Check sheet for the modelled part. Datum: model origin and axes. Units: mm. A direction names the side the tool comes from. Give positions to 0.01 mm unless a question says otherwise; leave off trailing zeros. Order: outer loops, then holes, each group sorted by start corner. A loop starts at its lowest first (then second) coordinate and runs counter-clockwise, first axis right, second up. Notation, with made-up numbers: (66.25, 23.25) -> (79.25, 23.25) arc R32 cw to (79.25, 59.25) -> close; hole circle Ø3 at (12, 57). An arc over 180 degrees is marked (long way). One line per question, with ' | ' between items. Start each with the question number.
from build123d import *

# Parameters (mm, degrees)
IZIM1_R                     = 5
Y_KSEKLIK_EKSTR_ZYON1_DEPTH = 20
IZIM1_3_R                   = 10
Y_KSEKLIK_EKSTR_ZYON2_DEPTH = 10
Y_KSEKLIK_EKSTR_ZYON3_DEPTH = 20


with BuildPart() as part:
    # izim1 → Y_kseklik-Ekstr_zyon1 (new body)
    with BuildSketch(Plane.XY):
        with BuildLine():
            ThreePointArc((0, 84.881835365), (-140.845, 0), (0, -84.881835365))
            ThreePointArc((0, -84.881835365), (140.845, 0), (0, 84.881835365))
        make_face()
        with Locations((-86.2825, 71.771855339)):
            Circle(IZIM1_R, mode=Mode.SUBTRACT)
        with Locations((-127.72, 0)):
            Circle(IZIM1_R, mode=Mode.SUBTRACT)
        with Locations((-116.616855339, -41.4375)):
            Circle(IZIM1_R, mode=Mode.SUBTRACT)
        with Locations((-86.2825, -71.771855339)):
            Circle(IZIM1_R, mode=Mode.SUBTRACT)
        with Locations((-44.845, -82.875)):
            Circle(IZIM1_R, mode=Mode.SUBTRACT)
        with Locations((86.2825, -71.771855339)):
            Circle(IZIM1_R, mode=Mode.SUBTRACT)
        with Locations((127.72, 0)):
            Circle(IZIM1_R, mode=Mode.SUBTRACT)
        with Locations((116.616855339, 41.4375)):
            Circle(IZIM1_R, mode=Mode.SUBTRACT)
        with Locations((86.2825, 71.771855339)):
            Circle(IZIM1_R, mode=Mode.SUBTRACT)
        with Locations((44.845, 82.875)):
            Circle(IZIM1_R, mode=Mode.SUBTRACT)
        with Locations((44.845, -82.875)):
            Circle(IZIM1_R, mode=Mode.SUBTRACT)
        with Locations((116.616855339, -41.4375)):
            Circle(IZIM1_R, mode=Mode.SUBTRACT)
        with Locations((-116.616855339, 41.4375)):
            Circle(IZIM1_R, mode=Mode.SUBTRACT)
        with Locations((-44.845, 82.875)):
            Circle(IZIM1_R, mode=Mode.SUBTRACT)
        with BuildLine():
            ThreePointArc((0, -53.422733691), (114.595, 0), (0, 53.422733691))
            ThreePointArc((0, 53.422733691), (-114.595, 0), (0, -53.422733691))
        make_face(mode=Mode.SUBTRACT)
    extrude(amount=Y_KSEKLIK_EKSTR_ZYON1_DEPTH)

    # izim1_3 → Y_kseklik-Ekstr_zyon2 (add)
    with BuildSketch(Plane.XY):
        with BuildLine():
            ThreePointArc((0, 53.422733691), (-114.595, 0), (0, -53.422733691))
            ThreePointArc((0, -53.422733691), (114.595, 0), (0, 53.422733691))
        make_face()
        with Locations((-44.845, 0)):
            Circle(IZIM1_3_R, mode=Mode.SUBTRACT)
        with Locations((44.845, 0)):
            Circle(IZIM1_3_R, mode=Mode.SUBTRACT)
    extrude(amount=Y_KSEKLIK_EKSTR_ZYON2_DEPTH)

    # izim1_5 → Y_kseklik-Ekstr_zyon3 (add)
    with BuildSketch(Plane.XY):
        with BuildLine():
            Line((44.845, 96), (-44.845, 96))
            ThreePointArc((-44.845, 96), (-21.743660159, 93.179011035), (0, 84.881835365))
            ThreePointArc((0, 84.881835365), (21.743660159, 93.179011035), (44.845, 96))
        make_face()
        with BuildLine():
            ThreePointArc((0, -84.881835365), (-21.743660159, -93.179011035), (-44.845, -96))
            Line((-44.845, -96), (44.845, -96))
            ThreePointArc((44.845, -96), (21.743660159, -93.179011035), (0, -84.881835365))
        make_face()
    extrude(amount=Y_KSEKLIK_EKSTR_ZYON3_DEPTH)


solid = part.part
1. Cross-section at C-C on x = -58. Record the boundary of the cut face in (y, z), and give its area (3 significant figures).
2. Scan lines: probe 1 along X at (y, z) = (0.5, 2.5); probe 2 along Y at (x, z) = (-84, 18.75); probe 3 along X at (y, z) = (-80.5, 3.5). Record each from-to range of solid material in increasing order.
3. Cross-section at D-D on z = 7. Give the number of separate pieces and of enclosed holes in the cut face, and give its area (3 significant figures).
4. Tool access check on faces 1 (the face through (-40.226, 80.96, 9.86)), 2 (the face through (-114.56, 2.22, 14.93)). Record the directions out of +Z, -Z, +X, -X, +Y, -Y that give a thin tool (end or side, any length) a straight path to the whole face; none if there is none.
5. Go/stop test with flat-tipped pins: pin 1 (6 mm diameter, centred on y = -54.5, z = 3.5, fed in from +X); pin 2 (5 mm diameter, centred on x = 52, z = 10.5, fed in from +Y); pin 3 (6 mm diameter, centred on x = 44.845, y = 82.875, fed in from +Z); pin 4 (1.5 mm diameter, centred on x = 46.5, y = -16.5, fed in from +Z). Record where each tip stops, or that it passes through.
6. Cross-section at A-A on y = 0. Record the boundary of the cut face in (x, z) (3 decimals).
7. Cross-section at B-B on x = 127.72. Record the boundary of the cut face in (y, z), and give its area (3 significant figures).
8. Mould release check, pull along Y, two halves, no side actions. Record for faces 3 (the face through (-1, -96, 10)), 4 (the face through (-111.848, -39.936, 9.86)), 5 (the face through (-140.82, 2.11, 9.86)): +Y half, -Y half, draft (parallel to the pull), parting line (faces both ways), or undercut.
Response values:
1) outline: (-95.09, 0) -> (95.09, 0) -> (95.09, 20) -> (68.5, 20) -> (68.5, 10) -> (-68.5, 10) -> (-68.5, 20) -> (-95.09, 20) -> close | area: 2,430 mm²
2) probe 1: x = -140.84 to -132.69, -122.75 to -54.83, -34.86 to 34.86, 54.83 to 122.75, 132.69 to 140.84 | probe 2: y = -87.65 to -76.22, -67.32 to -57.72, 57.72 to 67.32, 76.22 to 87.65 | probe 3: x = -97.15 to -49.24, -40.45 to 40.45, 49.24 to 97.15
3) separate pieces: 1 | enclosed holes: 16 | area: 44,400 mm²
4) face 1: +Z, -Z | face 2: +Z
5) pin 1: stops at x = 125.86 | pin 2: stops at y = 95.89 | pin 3: passes through | pin 4: stops at z = 10
6) outline: (-140.845, 0) -> (-132.72, 0) -> (-132.72, 20) -> (-140.845, 20) -> close; (-122.72, 0) -> (-54.845, 0) -> (-54.845, 10) -> (-114.595, 10) -> (-114.595, 20) -> (-122.72, 20) -> close; (-34.845, 0) -> (34.845, 0) -> (34.845, 10) -> (-34.845, 10) -> close; (54.845, 0) -> (122.72, 0) -> (122.72, 20) -> (114.595, 20) -> (114.595, 10) -> (54.845, 10) -> close; (132.72, 0) -> (140.845, 0) -> (140.845, 20) -> (132.72, 20) -> close
7) outline: (-48.45, 0) -> (-5, 0) -> (-5, 20) -> (-48.45, 20) -> close; (5, 0) -> (48.45, 0) -> (48.45, 20) -> (5, 20) -> close | area: 1,740 mm²
8) face 3: -Y half | face 4: undercut | face 5: parting line
